Model file for the job. Use its own axes, mm. A direction names the side the tool comes from. Coordinates: 2 decimals unless noted, no trailing zeros. Write each loop counter-clockwise with the first axis right and the second up, starting at its lowest first coordinate (ties: lowest second). Pieces come first, ordered by that corner, then holes. Notation, with made-up numbers: M 65,72.5 L 122,72.5 A34 ccw 122,109.5 Z; hole C -6.75,-24 d2. An arc over 180 degrees is marked long. Use CSV: the item, a comma, the result in double quotes. Start each with the question number.
from build123d import *

# Parameters (mm, degrees)
SKETCH1_W           = 47.244
SKETCH1_H           = 19.05
BOSS_EXTRUDE1_DEPTH = 7.62
SKETCH4_R           = 1.27
CUT_EXTRUDE3_DEPTH  = 7.62
SKETCH5_R           = 1.27
CUT_EXTRUDE4_DEPTH  = 7.62
CUT_EXTRUDE8_DEPTH  = 27.585501857


with BuildPart() as part:
    # Sketch1 → Boss-Extrude1 (new body)
    with BuildSketch(Plane(origin=(0, 0, 0), x_dir=(1, 0, 0), z_dir=(0, 1, 0))):
        Rectangle(SKETCH1_W, SKETCH1_H)
    extrude(amount=BOSS_EXTRUDE1_DEPTH)

    # Sketch4 → Cut-Extrude3 (cut)
    with BuildSketch(Plane(origin=(23.622, 0, 0), x_dir=(0, 0, -1), z_dir=(1, 0, 0))):
        with Locations((0, 3.786925891)):
            Circle(SKETCH4_R)
    extrude(amount=-CUT_EXTRUDE3_DEPTH, mode=Mode.SUBTRACT)

    # Sketch5 → Cut-Extrude4 (cut)
    with BuildSketch(Plane.ZY.offset(23.622)):
        with Locations((0, 3.81)):
            Circle(SKETCH5_R)
    extrude(amount=-CUT_EXTRUDE4_DEPTH, mode=Mode.SUBTRACT)

    # Sketch2 → Cut-Extrude8 (cut, through all)
    with BuildSketch(Plane(origin=(0, 7.62, 0), x_dir=(1, 0, 0), z_dir=(0, 1, 0))):
        Polygon((-17.272, 3.175), (-17.272, -3.175), (-6.166997771, 0), align=None)
        Polygon((17.272, 3.175), (6.1595, 0), (17.272, -3.175), align=None)
        Polygon((-17.272, 6.985), (-17.272, 6.694714286), (-0.005828805, 1.761522516), (17.272, 6.701378026), (17.272, 6.985), align=None)
        Polygon((-0.005828805, -1.761522516), (-17.272, -6.694714286), (-17.272, -6.985), (17.272, -6.985), (17.272, -6.701378026), align=None)
        Polygon((18.264007134, -6.985), (17.272, -6.701378026), (17.272, -6.985), align=None)
        Polygon((-17.272, -6.985), (-17.272, -6.694714286), (-18.288, -6.985), align=None)
        Polygon((-18.288, 6.985), (-17.272, 6.694714286), (-17.272, 6.985), align=None)
        Polygon((17.272, 6.985), (17.272, 6.701378026), (18.264007134, 6.985), align=None)
    extrude(amount=-CUT_EXTRUDE8_DEPTH, mode=Mode.SUBTRACT)


solid = part.part
1) Band-saw the part on C-C on y = 1.5. List the corners of the cut face in (x, z) (1 decimal), then the cut area to 3 significant figures.
2) Tool access for faces 5 (the face through (20.49, 2.55, 0.28)), 6 (the face through (0, 7.62, 0)), 7 (the face through (-20.49, 2.57, -0.28)), 8 (the face through (23.622, 5.4, 0.1)), 9 (the face through (-11.642, 3.863, -1.565)): list every direction of +Z, -Z, +X, -X, +Y, -Y with a clear straight run to the whole face (end or side of a thin tool).
3) Band-saw the part on D-D on x = 5.5. List the corners of the cut face in (y, z) (3 decimals), then the cut area to 3 significant figures.
4) Band-saw the part on B-B on x = -7.5. List the corners of the cut face in (y, z) (3 decimals).
5) Band-saw the part on A-A on z = 5.5. List the corners of the cut face in (x, y).
6) Two-plate mould, pull along X, no slides. Class faces 1 (the face through (-23.622, 5.4, 0.1)), 2 (the face through (0, 4, 9.525)), 3 (the face through (11.638, 3.863, 1.565)), 4 (the face through (0, 4, -6.985)): pulls with the +X half, pulls with the -X half, needs draft (parallel to the pull), parting line crosses it, or undercut.
7) Wall check: L1, parallel to Y at x = 20, z = 0; L2, parallel to Z at x = 7, y = 3.75 (3 decimals); L3, parallel to Z at x = -4, y = 5.25 (3 decimals). Give the ranges that are in metal, low to high. Write a range as [from, to].
Findings below:
1,outline,"M -23.6,-9.5 L 23.6,-9.5 L 23.6,9.5 L -23.6,9.5 Z; hole M -18.3,-7 L 18.3,-7 L 0,-1.8 Z; hole M -18.3,7 L 0,1.8 L 18.3,7 Z; hole M -17.3,-3.2 L -6.2,0 L -17.3,3.2 Z; hole M 6.2,0 L 17.3,-3.2 L 17.3,3.2 Z"
1,area,"639 mm2"
2,face 5,"+X"
2,face 6,"+Z, -Z, +X, -X, +Y"
2,face 7,"-X"
2,face 8,"+Z, -Z, +X, +Y, -Y"
2,face 9,"+Y, -Y"
3,outline,"M 0,-9.525 L 7.62,-9.525 L 7.62,-6.985 L 0,-6.985 Z; M 0,-3.336 L 7.62,-3.336 L 7.62,3.336 L 0,3.336 Z; M 0,6.985 L 7.62,6.985 L 7.62,9.525 L 0,9.525 Z"
3,area,"89.5 mm2"
4,outline,"M 0,-9.525 L 7.62,-9.525 L 7.62,-6.985 L 0,-6.985 Z; M 0,-3.903 L 7.62,-3.903 L 7.62,-0.381 L 0,-0.381 Z; M 0,0.381 L 7.62,0.381 L 7.62,3.903 L 0,3.903 Z; M 0,6.985 L 7.62,6.985 L 7.62,9.525 L 0,9.525 Z"
5,outline,"M -23.62,0 L -13.09,0 L -13.09,7.62 L -23.62,7.62 Z; M 13.07,0 L 23.62,0 L 23.62,7.62 L 13.07,7.62 Z"
6,face 1,"pulls with the -X half"
6,face 2,"needs draft"
6,face 3,"undercut"
6,face 4,"undercut"
7,L1,"y = [0, 2.52], [5.06, 7.62]"
7,L2,"z = [-9.525, -6.985], [-3.765, -0.24], [0.24, 3.765], [6.985, 9.525]"
7,L3,"z = [-9.525, -6.985], [-2.903, 2.903], [6.985, 9.525]"
